```python
from build123d import *

# Parameters (mm, degrees)
F0_W     = 37.6
F0_H     = 15.7
F1_DEPTH = 2.2
F3_DEPTH = 0.25
F4_W     = 2.5
F4_H     = 15.7
F5_DEPTH = 2
F6_W     = 8
F6_H     = 8
F6_W_2   = 6.5
F7_DEPTH = 1


with BuildPart() as f1:
    # F0 (on Top) → F1 (new body)
    with BuildSketch(Plane.XY):
        Rectangle(F0_W, F0_H)
    extrude(amount=F1_DEPTH)

    # F2 (on face) → F3 (join)
    with BuildSketch(Plane.XY.offset(2.2)):
        Polygon((17.908588, 6), (17.408588, 6), (17.408588, 5.5), (14.708588, 5.5), (14.708588, 4), (15.208588, 4), (17.408588, 4), (17.408588, 3.5), (14.708588, 3.5), (14.708588, 2), (17.408588, 2), (17.408588, 1.5), (14.708588, 1.5), (14.708588, 0), (17.408588, 0), (17.408588, -0.5), (14.708588, -0.5), (14.708588, -2), (17.408588, -2), (17.408588, -2.5), (14.708588, -2.5), (14.708588, -4), (17.408588, -4), (17.408588, -4.5), (14.708588, -4.5), (14.708588, -6), (17.908588, -6), (17.908588, -5.5), (15.208588, -5.5), (15.208588, -5), (17.908588, -5), (17.908588, -3.5), (15.208588, -3.5), (15.208588, -3), (17.908588, -3), (17.908588, -1.5), (15.208588, -1.5), (15.208588, -1), (17.908588, -1), (17.908588, 0.5), (15.208588, 0.5), (15.208588, 1), (17.908588, 1), (17.908588, 2.5), (15.208588, 2.5), (15.208588, 3), (17.908588, 3), (17.908588, 4.5), (15.208588, 4.5), (15.208588, 5), (17.908588, 5), align=None)
    extrude(amount=F3_DEPTH)

    # F4 (on face) → F5 (join)
    with BuildSketch(Plane.XY.offset(2.2)):
        with Locations((-17.55, 0)):
            Rectangle(F4_W, F4_H)
    extrude(amount=F5_DEPTH)

    # F6 (on face) → F7 (join)
    with BuildSketch(Plane.XY.offset(2.2)):
        with Locations((-4.5, 1.85)):
            Rectangle(F6_W, F6_H)
        with Locations((3.75, 1.85)):
            Rectangle(F6_W_2, F6_H)
    extrude(amount=F7_DEPTH)


solid = f1.part
```
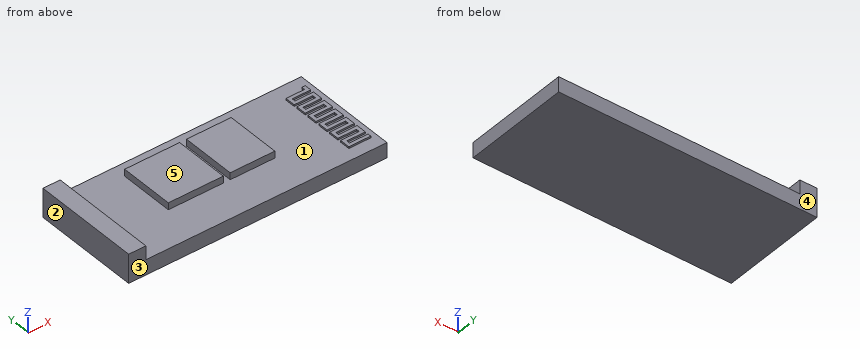
Verification items for the finished model (mm, model axes). Face numbers are marked on the shaded views. A direction names the side the tool comes from. Round coordinates to 2 decimals unless told otherwise and drop trailing zeros. Write each loop counter-clockwise with the first axis right and the second up, starting at its lowest first coordinate (ties: lowest second). Pieces come first, ordered by that corner, then holes.
1. Section check A-A on x = -1.5. Enter the section's corners in (y, z).
2. Draft check along X on the marked faces 1, 2 and 3. Enter one of: +X half, -X half, draft (parallel to the pull), parting line (faces both ways), or undercut.
3. Section check B-B on x = 13. Enter the section's corners in (y, z).
4. Access from +Z, -Z, +X, -X, +Y, -Y to the whole of each face (thin tool, end or side, straight path). Record for the marked faces 4 and 5.
5. Gauge pin test, flat ends, axial feed: P1, Ø2, axis at x = -4.5, y = -4.5, coming from the +Z side; P2, Ø1.5, axis at y = 5, z = 3.5, coming from the +X side; P3, Ø1, axis at x = -4, y = 4, coming from the +Z side. Record the tip position at first contact, or that the pin passes through.
6. Scan lines: L1, parallel to X at y = 4, z = 3.1; L2, parallel to Z at x = 8, y = 0.5; L3, parallel to X at y = -1.5, z = 3.25. Record each from-to range of solid material in increasing order.
Answer:
1. outline: (-7.85, 0) - (7.85, 0) - (7.85, 2.2) - (5.85, 2.2) - (5.85, 3.2) - (-2.15, 3.2) - (-2.15, 2.2) - (-7.85, 2.2) - close
2. face 1: undercut
2. face 2: -X half
2. face 3: draft
3. outline: (-7.85, 0) - (7.85, 0) - (7.85, 2.2) - (-7.85, 2.2) - close
4. face 4: +Z, -Z, +X, -X, +Y
4. face 5: +Z, +X, +Y, -Y
5. P1: stops at z = 2.2
5. P2: stops at x = 7
5. P3: stops at z = 3.2
6. L1: x = -18.8 to -16.3, -8.5 to -0.5, 0.5 to 7
6. L2: z = 0 to 2.2
6. L3: x = -18.8 to -16.3
